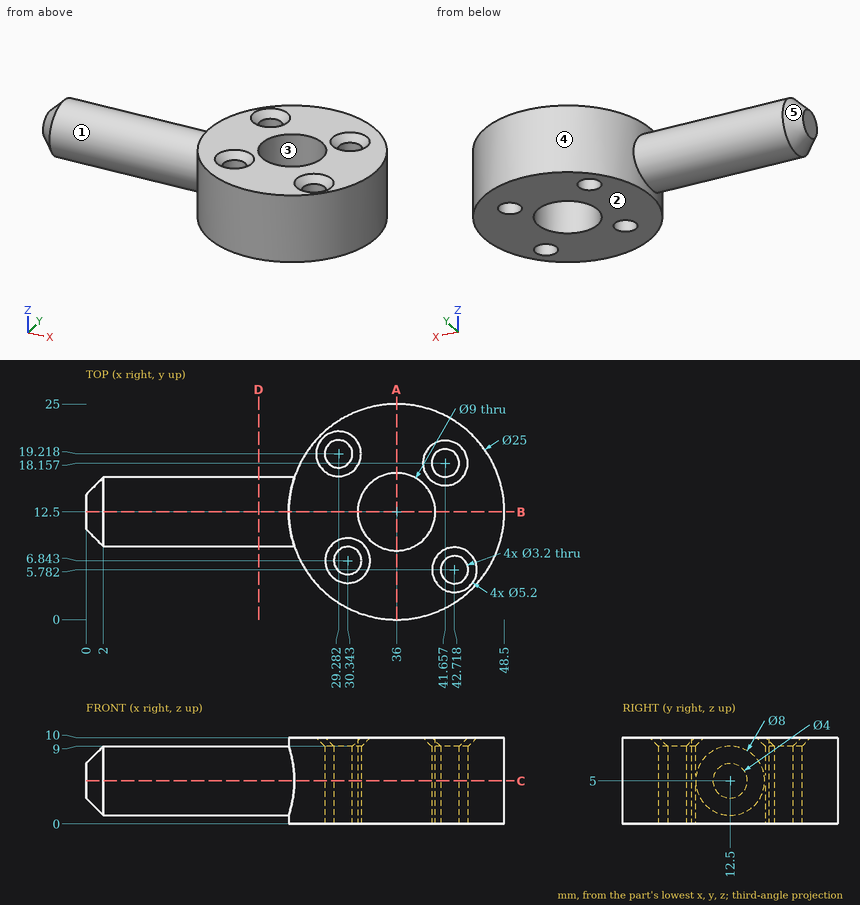
Answer from the drawing. Dimensions are ordinates in mm from the lowest x, y and z of the part. A direction names the side the tool comes from. Coordinates: 2 decimals unless noted, no trailing zeros. Loops run counter-clockwise (first coordinate to the right, second up) from the corner with the lowest first, then second, coordinate; pieces in that order, holes last.
1) Section B-B (y = 12.5) is taken. Give the vertices of the cut face in (x, z).
Results:
outline: (0, 3) - (2, 1) - (23.5, 1) - (23.5, 0) - (31.5, 0) - (31.5, 10) - (23.5, 10) - (23.5, 9) - (2, 9) - (0, 7) - close; (40.5, 0) - (48.5, 0) - (48.5, 10) - (40.5, 10) - close
2) Section D-D (x = 20) is taken. Give the vertices of the cut face in (y, z).
Results:
outline: circle Ø8 at (12.5, 5)
3) For the marked faces 1 and 2, determine the directions among +Z, -Z, +X, -X, +Y, -Y from which every point of the face is accessible in a straight line to the end or side of a thin tool.
Results:
face 1: -X
face 2: -Z, +X, -X, +Y, -Y
4) For a pull along X with two mould halves and no side action, classify the marked faces 3, 4 and 5 as +X half, -X half, draft (parallel to the pull), parting line (faces both ways), or undercut.
Results:
face 3: undercut
face 4: parting line
face 5: -X half
5) Section C-C (z = 5) is taken. Give the vertices of the cut face in (x, y), plus the area to 3 significant figures.
Results:
outline: (0, 10.5) - (2, 8.5) - (24.16, 8.5) arc R12.5 ccw (long way) to (24.16, 16.5) - (2, 16.5) - (0, 14.5) - close; hole circle Ø3.2 at (29.28, 19.22); hole circle Ø3.2 at (30.34, 6.84); hole circle Ø9 at (36, 12.5); hole circle Ø3.2 at (41.66, 18.16); hole circle Ø3.2 at (42.72, 5.78)
area: 581 mm2
6) Consider probe 1 along Y at (x, z) = (42, 0.5) (1 decimal); probe 2 along Y at (x, z) = (34.5, 9.25); probe 3 along X at (y, z) = (11, 5.5). Determine where each line is inside the solid, lowest interval first.
Results:
probe 1: y = 1.5 to 4.4, 7.2 to 16.6, 19.7 to 23.5
probe 2: y = 0.09 to 8.26, 16.74 to 24.91
probe 3: x = 0 to 31.76, 40.24 to 48.41
7) Section A-A (x = 36) is taken. Give the vertices of the cut face in (y, z).
Results:
outline: (0, 0) - (8, 0) - (8, 10) - (0, 10) - close; (17, 0) - (25, 0) - (25, 10) - (17, 10) - close
8) Flat-ended cylindrical pins translate along their axes: pin 1 (5 mm diameter, centred on x = 41.66, y = 18.16, fed in from +Z) (1 decimal); pin 2 (1.5 mm diameter, centred on x = 6, z = 6.5, fed in from -Y); pin 3 (3 mm diameter, centred on y = 19, z = 5.5, fed in from +X); pin 4 (10.5 mm diameter, centred on x = 36, y = 12.5, fed in from -Z). Find the tip coordinate at first contact, or state that the pin passes through.
Results:
pin 1: stops at z = 9.9
pin 2: stops at y = 8.57
pin 3: stops at x = 47.46
pin 4: stops at z = 0
